Job drawing, mm, ordinate dimensions from the low corner. One solid piece. A direction names the side the tool comes from. Give positions to 0.01 mm unless a question says otherwise; leave off trailing zeros. Order: outer loops, then holes, each group sorted by start corner. A loop starts at its lowest first (then second) coordinate and runs counter-clockwise, first axis right, second up. Notation, with made-up numbers: (67.25, 33.5) - (120.25, 33.5) arc R22 cw to (120.25, 60.5) - close; hole circle Ø5 at (61, 8.5). An arc over 180 degrees is marked (long way). Use one line per item in the form item = value. Start each with the question number.
1. Band-saw the part on D-D, the plane z = 2.5. List the corners of the cut face in (x, y) (3 decimals).
2. Band-saw the part on C-C, the plane z = 5.5. List the corners of the cut face in (x, y).
3. Drill centre lines: line 1 (Z direction, x = 1, y = 17); line 2 (Y direction, x = 13, z = 5.7); line 3 (Y direction, x = 13, z = 2.3) (3 decimals). Where is each one in solid material? Low to high.
4. Tool access for the marked faces 1, 2 and 3: list every direction of +Z, -Z, +X, -X, +Y, -Y with a clear straight run to the whole face (end or side of a thin tool).
5. Pin check, flat tips, straight feed: P1, Ø5.5, axis at x = 13, y = 13, coming from the +Z side; P2, Ø1.5, axis at x = 9.5, z = 4, coming from the +Y side; P3, Ø4, axis at x = 9.5, z = 6, coming from the +Y side. Stop position of each tip, or through.
6. Band-saw the part on A-A, the plane y = 13. List the corners of the cut face in (x, z).
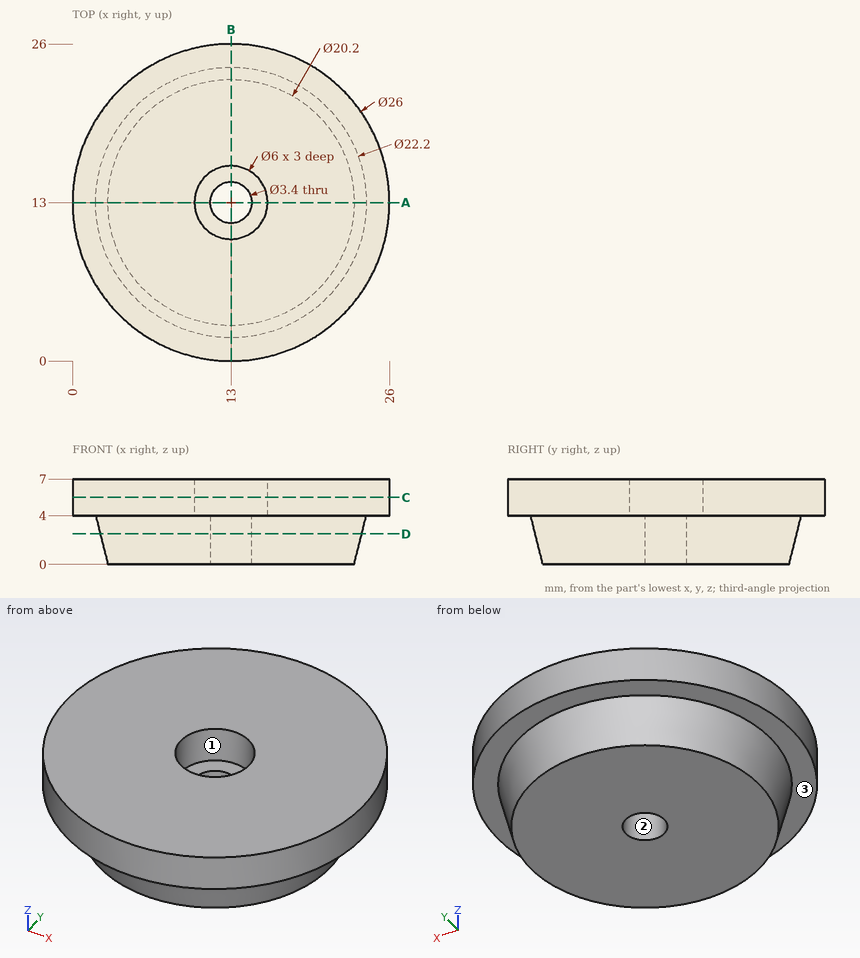
From the geometry:
q1.outline = circle Ø21.45 at (13, 13); hole circle Ø3.4 at (13, 13)
q2.outline = circle Ø26 at (13, 13); hole circle Ø6 at (13, 13)
q3.line_1 = 4 to 7
q3.line_2 = 0 to 10, 16 to 26
q3.line_3 = 2.325 to 11.3, 14.7 to 23.675
q4.face_1 = +Z
q4.face_2 = +Z, -Z
q4.face_3 = -Z
q5.P1 = 4
q5.P2 = 25.71
q5.P3 = 25.91
q6.outline = (0, 4) - (1.9, 4) - (2.9, 0) - (11.3, 0) - (11.3, 4) - (10, 4) - (10, 7) - (0, 7) - close; (14.7, 0) - (23.1, 0) - (24.1, 4) - (26, 4) - (26, 7) - (16, 7) - (16, 4) - (14.7, 4) - close
